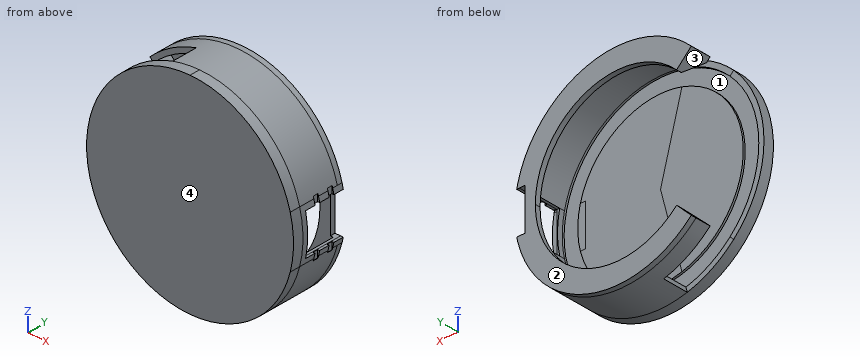
from build123d import *
from build123d.topology import SkipClean

# Parameters (mm, degrees)
SKETCH1_R            = 100
BOSS_EXTRUDE1_DEPTH  = 10
SKETCH2_R            = 95
SKETCH2_R_2          = 80
CUT_EXTRUDE1_DEPTH   = 2
BOSS_EXTRUDE2_DEPTH  = 40
BOSS_EXTRUDE3_DEPTH  = 5
CUT_EXTRUDE2_START   = -5
SKETCH5_W            = 50
SKETCH5_H            = 40
CUT_EXTRUDE2_DEPTH   = 40
BOSS_EXTRUDE4_START  = -45
BOSS_EXTRUDE4_DEPTH  = 45
SKETCH8_W            = 40
SKETCH8_H            = 5
BOSS_EXTRUDE5_DEPTH  = 55
CUT_EXTRUDE3_START   = -10
SKETCH10_W           = 8.429508811
SKETCH10_H           = 40
CUT_EXTRUDE3_DEPTH   = 10
BOSS_EXTRUDE6_START  = 18.2
BOSS_EXTRUDE6_DEPTH  = 2
BOSS_EXTRUDE7_START  = 18.1
BOSS_EXTRUDE7_DEPTH  = 15
SKETCH13_W           = 20.653307815
SKETCH13_H           = 40
CUT_EXTRUDE4_DEPTH   = 5
BOSS_EXTRUDE8_DEPTH  = 17
BOSS_EXTRUDE9_DEPTH  = 3
BOSS_EXTRUDE10_DEPTH = 3
SKETCH18_W           = 11.98170237
SKETCH18_H           = 40
CUT_EXTRUDE5_DEPTH   = 5
CUT_EXTRUDE6_START   = -20
CUT_EXTRUDE6_DEPTH   = 25
CUT_EXTRUDE7_START   = -200
CUT_EXTRUDE7_DEPTH   = 200
CUT_EXTRUDE8_DEPTH   = 40
CUT_EXTRUDE9_START   = 6
SKETCH23_W           = 7
SKETCH23_H           = 5
CUT_EXTRUDE9_DEPTH   = 40


with BuildPart() as part:
    # Sketch1 → Boss-Extrude1 (new body)
    with BuildSketch(Plane(origin=(0, 0, 0), x_dir=(1, 0, 0), z_dir=(0, 1, 0))):
        with Locations(Location((0, 0, 0), (0, 0, 270))):
            Circle(SKETCH1_R)
    extrude(amount=BOSS_EXTRUDE1_DEPTH)

    # Sketch2 → Cut-Extrude1 (cut)
    with BuildSketch(Plane(origin=(0, 10, 0), x_dir=(1, 0, 0), z_dir=(0, 1, 0))):
        with Locations(Location((0, 0, 0), (0, 0, 270))):
            Circle(SKETCH2_R)
        with Locations(Location((0, 0, 0), (0, 0, 270))):
            Circle(SKETCH2_R_2, mode=Mode.SUBTRACT)
    extrude(amount=-CUT_EXTRUDE1_DEPTH, mode=Mode.SUBTRACT)

    # Sketch3 → Boss-Extrude2 (add)
    with SkipClean():  # the faces are left unmerged after this step: merging them gives an invalid solid
        with BuildSketch(Plane(origin=(0, 10, 0), x_dir=(1, 0, 0), z_dir=(0, 1, 0))):
            with BuildLine():
                Line((-67.175144213, 67.175144213), (-70.710678119, 70.710678119))
                ThreePointArc((-70.710678119, 70.710678119), (100, 0), (-70.710678119, -70.710678119))
                Line((-70.710678119, -70.710678119), (-67.175144213, -67.175144213))
                ThreePointArc((-67.175144213, -67.175144213), (95, 0), (-67.175144213, 67.175144213))
            make_face()
        extrude(amount=BOSS_EXTRUDE2_DEPTH)

    # Sketch5 → Cut-Extrude2 (cut)
    with SkipClean():  # the faces are left unmerged after this step: merging them gives an invalid solid
        with BuildSketch(Plane(origin=(0, 55, 0), x_dir=(1, 0, 0), z_dir=(0, 1, 0)).offset(CUT_EXTRUDE2_START)):
            with Locations((102.459666924, 0)):
                Rectangle(SKETCH5_W, SKETCH5_H)
        extrude(amount=-CUT_EXTRUDE2_DEPTH, mode=Mode.SUBTRACT)



with BuildPart() as body_2:
    # Sketch4 → Boss-Extrude3 (new body)
    with BuildSketch(Plane(origin=(0, 50, 0), x_dir=(1, 0, 0), z_dir=(0, 1, 0))):
        with BuildLine():
            ThreePointArc((-67.175144213, -67.175144213), (95, 0), (-67.175144213, 67.175144213))
            Line((-67.175144213, 67.175144213), (-56.568542495, 56.568542495))
            ThreePointArc((-56.568542495, 56.568542495), (30.614674589, 73.910362601), (80, 0))
            ThreePointArc((80, 0), (30.614674589, -73.910362601), (-56.568542495, -56.568542495))
            Line((-56.568542495, -56.568542495), (-67.175144213, -67.175144213))
        make_face()
        with BuildLine():
            Line((-70.710678119, 70.710678119), (-67.175144213, 67.175144213))
            ThreePointArc((-67.175144213, 67.175144213), (95, 0), (-67.175144213, -67.175144213))
            Line((-67.175144213, -67.175144213), (-70.710678119, -70.710678119))
            ThreePointArc((-70.710678119, -70.710678119), (100, 0), (-70.710678119, 70.710678119))
        make_face()
    extrude(amount=BOSS_EXTRUDE3_DEPTH)


with BuildPart() as part_1:
    with SkipClean():  # the faces are left unmerged after this step: merging them gives an invalid solid
        add(part.part)

        add(body_2.part)  # Boss-Extrude4 merges body 2
        # Sketch7 → Boss-Extrude4 (add)
        with BuildSketch(Plane(origin=(0, 55, 0), x_dir=(1, 0, 0), z_dir=(0, 1, 0)).offset(BOSS_EXTRUDE4_START)):
            with BuildLine():
                ThreePointArc((96.824583655, 25), (97.434164903, 22.507410108), (97.979589711, 20))
                Line((97.979589711, 20), (127.459666924, 20))
                Line((127.459666924, 20), (127.459666924, -20))
                Line((127.459666924, -20), (97.979589711, -20))
                ThreePointArc((97.979589711, -20), (97.434164903, -22.507410108), (96.824583655, -25))
                Line((96.824583655, -25), (132.459666924, -25))
                Line((132.459666924, -25), (132.459666924, 25))
                Line((132.459666924, 25), (96.824583655, 25))
            make_face()
        extrude(amount=BOSS_EXTRUDE4_DEPTH)

    # Sketch8 → Boss-Extrude5 (add)
    with SkipClean():  # the faces are left unmerged after this step: merging them gives an invalid solid
        with BuildSketch(Plane.ZY.offset(-127.459666924)):
            with Locations((0, 12.5)):
                Rectangle(SKETCH8_W, SKETCH8_H)
        extrude(amount=BOSS_EXTRUDE5_DEPTH)

    # Sketch10 → Cut-Extrude3 (cut)
    with SkipClean():  # the faces are left unmerged after this step: merging them gives an invalid solid
        with BuildSketch(Plane.XZ.offset(CUT_EXTRUDE3_START)):
            with Locations((88.6561237, 0)):
                Rectangle(SKETCH10_W, SKETCH10_H)
            with BuildLine():
                Line((92.870878105, -20), (92.870878105, 20))
                ThreePointArc((92.870878105, 20), (95, 0), (92.870878105, -20))
            make_face()
        extrude(amount=-CUT_EXTRUDE3_DEPTH, mode=Mode.SUBTRACT)

    # Sketch13 → Cut-Extrude4 (cut)
    with SkipClean():  # the faces are left unmerged after this step: merging them gives an invalid solid
        with BuildSketch(Plane(origin=(0, 55, 0), x_dir=(1, 0, 0), z_dir=(0, 1, 0))):
            with Locations((100.326653908, 0)):
                Rectangle(SKETCH13_W, SKETCH13_H)
        extrude(amount=-CUT_EXTRUDE4_DEPTH, mode=Mode.SUBTRACT)



with BuildPart() as body_2_2:
    # Sketch11 → Boss-Extrude6 (new body)
    with BuildSketch(Plane(origin=(0, 15, 0), x_dir=(1, 0, 0), z_dir=(0, 1, 0)).offset(BOSS_EXTRUDE6_START)):
        with BuildLine():
            Line((110.459666924, 8), (95.459666924, 8))
            Line((95.459666924, 8), (95.459666924, 3.5))
            Line((95.459666924, 3.5), (100.359666924, 3.5))
            ThreePointArc((100.359666924, 3.5), (103.859666924, 0), (100.359666924, -3.5))
            Line((100.359666924, -3.5), (95.459666924, -3.5))
            Line((95.459666924, -3.5), (95.459666924, -8))
            Line((95.459666924, -8), (110.459666924, -8))
            Line((110.459666924, -8), (110.459666924, 8))
        make_face()
    extrude(amount=BOSS_EXTRUDE6_DEPTH)

    # Sketch12 → Boss-Extrude7 (add)
    with BuildSketch(Plane(origin=(0, 15, 0), x_dir=(1, 0, 0), z_dir=(0, 1, 0)).offset(BOSS_EXTRUDE7_START)):
        Polygon((95.459666924, -10), (95.459666924, -8), (110.459666924, -8), (110.459666924, 8), (95.459666924, 8), (95.459666924, 10), (112.459666924, 10), (112.459666924, -10), align=None)
    extrude(amount=BOSS_EXTRUDE7_DEPTH)


with BuildPart() as part_2:
    with SkipClean():  # the faces are left unmerged after this step: merging them gives an invalid solid
        add(part_1.part)

        add(body_2_2.part)  # Boss-Extrude8 merges body 2 2
        # Sketch15 → Boss-Extrude8 (add)
        with BuildSketch(Plane(origin=(112.459666924, 0, 0), x_dir=(0, 0, -1), z_dir=(1, 0, 0))):
            Polygon((-8.249409199, 33.1), (-18.249409392, 15), (-20, 15), (-20, 15.967177607), (-10, 34.067177257), align=None)
            Polygon((10, 34.067177257), (20, 15.967177607), (20, 15), (18.249409392, 15), (8.249409199, 33.1), align=None)
        extrude(amount=-BOSS_EXTRUDE8_DEPTH)

    # Sketch16 → Boss-Extrude9 (add)
    with BuildSketch(Plane(origin=(0, 0, 0), x_dir=(0.7071067811865464, 0, 0.7071067811865487), z_dir=(-0.7071067811865487, 0, 0.7071067811865464))):
        Polygon((-80, 50), (-95, 35), (-95, 50), align=None)
    extrude(amount=-BOSS_EXTRUDE9_DEPTH)

    # Sketch17 → Boss-Extrude10 (add)
    with BuildSketch(Plane(origin=(0, 0, 0), x_dir=(-0.7071067811865475, 0, 0.7071067811865477), z_dir=(-0.7071067811865477, 0, -0.7071067811865475))):
        Polygon((80, 50), (95, 35), (95, 50), align=None)
    extrude(amount=-BOSS_EXTRUDE10_DEPTH)

    # Sketch18 → Cut-Extrude5 (cut)
    with BuildSketch(Plane(origin=(0, 15, 0), x_dir=(1, 0, 0), z_dir=(0, 1, 0))):
        with Locations((78.450518109, 0)):
            Rectangle(SKETCH18_W, SKETCH18_H)
    extrude(amount=-CUT_EXTRUDE5_DEPTH, mode=Mode.SUBTRACT)

    # Sketch20 → Cut-Extrude6 (cut)
    with BuildSketch(Plane(origin=(0, 55, 0), x_dir=(1, 0, 0), z_dir=(0, 1, 0)).offset(CUT_EXTRUDE6_START)):
        with BuildLine():
            Line((0, 0), (-31.757481462, 118.520534337))
            ThreePointArc((-31.757481462, 118.520534337), (-122.701486088, 0), (-31.757481462, -118.520534337))
            Line((-31.757481462, -118.520534337), (0, 0))
        make_face()
    extrude(amount=-CUT_EXTRUDE6_DEPTH, mode=Mode.SUBTRACT)

    # Sketch21 → Cut-Extrude7 (cut)
    with BuildSketch(Plane(origin=(0, 55, 0), x_dir=(1, 0, 0), z_dir=(0, 1, 0)).offset(CUT_EXTRUDE7_START)):
        with BuildLine():
            Line((96.824583655, 25), (132.459666924, 25))
            Line((132.459666924, 25), (132.459666924, -25))
            Line((132.459666924, -25), (96.824583655, -25))
            ThreePointArc((96.824583655, -25), (100, 0), (96.824583655, 25))
        make_face()
    extrude(amount=CUT_EXTRUDE7_DEPTH, mode=Mode.SUBTRACT)

    # Sketch22 → Cut-Extrude8 (cut)
    with BuildSketch(Plane(origin=(0, 55, 0), x_dir=(1, 0, 0), z_dir=(0, 1, 0))):
        Polygon((95.459666924, 20), (95.459666924, -20), (121.621169639, -20), (97.979589711, 20), align=None)
    extrude(amount=-CUT_EXTRUDE8_DEPTH, mode=Mode.SUBTRACT)

    # Sketch23 → Cut-Extrude9 (cut)
    with SkipClean():  # the faces are left unmerged after this step: merging them gives an invalid solid
        with BuildSketch(Plane(origin=(90, 0, 0), x_dir=(0, 0, -1), z_dir=(1, 0, 0)).offset(CUT_EXTRUDE9_START)):
            with Locations((-23.5, 42.5)):
                Rectangle(SKETCH23_W, SKETCH23_H)
            with Locations((-23.5, 27.5)):
                Rectangle(SKETCH23_W, SKETCH23_H)
            with Locations((23.5, 27.5)):
                Rectangle(SKETCH23_W, SKETCH23_H)
            with Locations((23.5, 42.5)):
                Rectangle(SKETCH23_W, SKETCH23_H)
        extrude(amount=CUT_EXTRUDE9_DEPTH, mode=Mode.SUBTRACT)


solid = part_2.part
Read the model definition and answer for the solid it produces. Units are mm, in the model's axes. Face numbers are marked on the shaded views. A direction names the side the tool comes from. Coordinates: 2 decimals unless noted, no trailing zeros. Write each loop counter-clockwise with the first axis right and the second up, starting at its lowest first coordinate (ties: lowest second). Pieces come first, ordered by that corner, then holes. Notation, with made-up numbers: M 53.25,46 L 71.25,46 A16 cw 71.25,60 Z; hole C 58.25,-8.5 d1. An arc over 180 degrees is marked long. Use a Markdown table: item, result.
Q1. Determine the mould class of the marked faces 1 and 2 for opening direction Z: released by +Z, released by -Z, zero draft, split by the parting line, or undercut.
Answer block:
| item | result |
|---|---|
| face 1 | undercut |
| face 2 | zero draft |
Q2. Each of these flat-tipped pins is pushed along its axis until it touches: pin 1 Ø8 at (x, z) = (58, -18.5) entering from +Y; pin 2 Ø2.5 at (y, z) = (43.5, -24.5) entering from +X; pin 3 Ø9 at (x, z) = (-39.5, -87) entering from -Y; pin 4 Ø1.4 at (x, z) = (97, 5) entering from +Y. Where does it stop, or does it pass through?
Answer block:
| item | result |
|---|---|
| pin 1 | stops at y = 10 |
| pin 2 | stops at x = 96 |
| pin 3 | stops at y = 0 |
| pin 4 | stops at y = 15 |
Q3. Which of the six approach directions +Z, -Z, +X, -X, +Y, -Y give full straight-line access (tool end or side, diameter ignored) to the marked faces 3 and 4?
Answer block:
| item | result |
|---|---|
| face 3 | -X, +Y |
| face 4 | +Z, -Z, +X, -X, -Y |
Q4. The part is cut by section B-B, the plane x = 49.5. Write down the section's boundary in (y, z), then the cut area to 3 significant figures.
Answer block:
| item | result |
|---|---|
| outline | M 0,-86.89 L 55,-86.89 L 55,-62.85 L 50,-62.85 L 50,-81.08 L 8,-81.08 L 8,-62.85 L 10,-62.85 L 10,62.85 L 8,62.85 L 8,81.08 L 50,81.08 L 50,62.85 L 55,62.85 L 55,86.89 L 0,86.89 Z |
| area | 2,370 mm2 |
Q5. Straight lines are drawn through the part: L1, parallel to Z at x = 0, y = 8.85; L2, parallel to Z at x = -0.5, y = 25.5. For each, find the intervals that lie inside material, in ascending order. Write a range as [from, to].
Answer block:
| item | result |
|---|---|
| L1 | z = [-100, -95], [-80, 80], [95, 100] |
| L2 | z = [-100, -95], [95, 100] |
Q6. The part is cut by section A-A, the plane x = 24. Write down the section's boundary in (y, z).
Answer block:
| item | result |
|---|---|
| outline | M 0,-97.08 L 55,-97.08 L 55,-76.32 L 50,-76.32 L 50,-91.92 L 8,-91.92 L 8,-76.32 L 10,-76.32 L 10,76.32 L 8,76.32 L 8,91.92 L 50,91.92 L 50,76.32 L 55,76.32 L 55,97.08 L 0,97.08 Z |
